Study the drawing (mm; zero at the part's minimum x, y, z) and answer. Round coordinates to 2 decimals unless told otherwise and drop trailing zeros. Order: outer loops, then holes, each group sorted by start corner. A loop starts at its lowest first (then second) coordinate and runs counter-clockwise, first axis right, second up. Notation, with made-up numbers: (-24, -38.75) - (-17, -38.75) arc R11 ccw to (-17, -34.75) - close; hole circle Ø2 at (32.25, 40.5). An arc over 180 degrees is marked (long way). Use one line per item in the form item = value. Start each with the question number.
Q1. The part is cut by section D-D on y = 21. Determine the outline of the cut face in (x, z).
Q2. The part is cut by section C-C on x = 84. Determine the outline of the cut face in (y, z) (3 decimals).
Q3. The part is cut by section B-B on z = 6.35. Determine the outline of the cut face in (x, y) (3 decimals), plus the area to 3 significant figures.
Q4. Find the intervals of material crossed by line 1 (X direction, y = 15.5, z = 7.75); line 2 (X direction, y = 10.75, z = 11.75); line 3 (X direction, y = 1.25, z = 9), in increasing order. Write a range as [from, to].
Q5. Given P1, Ø8, axis at x = 177.5, y = 10.5, coming from the +Z side (3 decimals); P2, Ø4, axis at x = 23, y = 16.5, coming from the -Z side; P3, Ø12, axis at x = 76, y = 19.5, coming from the +Z side, each flat-ended and moving along its own axis, determine where each tip first touches the part or whether it passes through.
Q6. The part is cut by section A-A on y = 12.7. Determine the outline of the cut face in (x, z) (3 decimals).
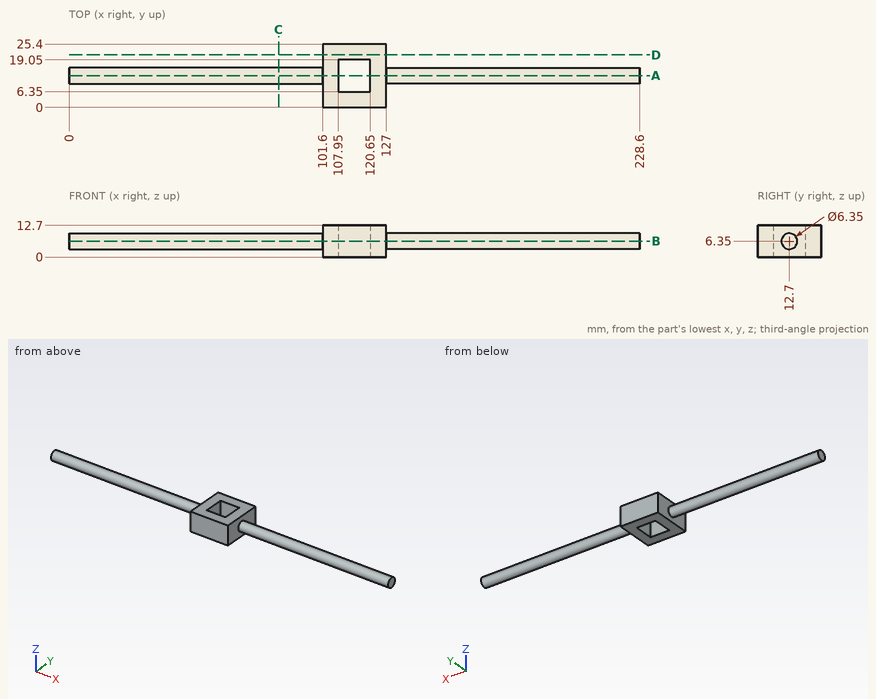
Found:
q1.outline = (101.6, 0) - (127, 0) - (127, 12.7) - (101.6, 12.7) - close
q2.outline = circle Ø6.35 at (12.7, 6.35)
q3.outline = (0, 9.525) - (101.6, 9.525) - (101.6, 0) - (127, 0) - (127, 9.525) - (228.6, 9.525) - (228.6, 15.875) - (127, 15.875) - (127, 25.4) - (101.6, 25.4) - (101.6, 15.875) - (0, 15.875) - close; hole (107.95, 6.35) - (120.65, 6.35) - (120.65, 19.05) - (107.95, 19.05) - close
q3.area = 1,770 mm²
q4.line_1 = [0, 107.95], [120.65, 228.6]
q4.line_2 = [101.6, 107.95], [120.65, 127]
q4.line_3 = [101.6, 127]
q5.P1 = 9.525
q5.P2 = 3.73
q5.P3 = 9.42
q6.outline = (0, 3.175) - (101.6, 3.175) - (101.6, 0) - (107.95, 0) - (107.95, 12.7) - (101.6, 12.7) - (101.6, 9.525) - (0, 9.525) - close; (120.65, 0) - (127, 0) - (127, 3.175) - (228.6, 3.175) - (228.6, 9.525) - (127, 9.525) - (127, 12.7) - (120.65, 12.7) - close
